Autodesk Inventor part; units mm, degrees
ref_plane "YZ Plane" through (0, 0, 0) normal (1, 0, 0) x (0, 1, 0)
ref_plane "XZ Plane" through (0, 0, 0) normal (0, 1, 0) x (-1, 0, 0)
ref_plane "XY Plane" through (0, 0, 0) normal (0, 0, 1) x (1, 0, 0)
sketch "Szkic1" plane through (0, 0, 0) normal (0, 0, 1) x (1, 0, 0)
  line L0 (3.7528, 6.5) -> (7.5056, 0)
  line L1 (7.5056, 0) -> (3.7528, -6.5)
  line L2 (3.7528, -6.5) -> (-3.7528, -6.5)
  line L3 (-3.7528, -6.5) -> (-7.5056, 0)
  line L4 (-7.5056, 0) -> (-3.7528, 6.5)
  line L5 (-3.7528, 6.5) -> (3.7528, 6.5)
  point P0 (0, 0)
  point P1 (0, 0)
  point P2 (0, 6.5)
extrude "Wyciągnięcie proste1" add sketch "Szkic1" along normal blind 5.5
sketch "Szkic2" plane through (0, 0, 5.5) normal (0, 0, 1) x (1, 0, 0)
  circle A0 centre (0, 0) radius 4
  dimension "d3" = 8
extrude "Wyciągnięcie proste2" add sketch "Szkic2" along normal blind 20
sketch "Szkic3" plane through (0, 0, 25.5) normal (0, 0, 1) x (1, 0, 0)
  circle A0 centre (0, 0) radius 4
  circle A1 centre (0, 0) radius 3.675
  dimension "d6" = 7.35
extrude "Wyciągnięcie proste3" add sketch "Szkic3" along normal blind 5 contours A1
sketch "Szkic4" plane through (0, 0, 30.5) normal (0, 0, 1) x (1, 0, 0)
  circle A0 centre (0, 0) radius 4
extrude "Wyciągnięcie proste4" add sketch "Szkic4" along normal blind 35
thread "Gwint1"
fillet "Zaokrąglenie1" radius 2 2 edges at (-3.675, 0, 25.5) (-3.675, 0, 30.5)
chamfer "Faza1" distance 0.5 angle 45 1 edges at (-4, 0, 65.5)
properties part number "COTS_GENERIC_M8_Hobbed_Bolt"
For this review, take the finished solid that the model builds, in its own axes (mm). A direction names the side the tool comes from. Round coordinates to 2 decimals unless told otherwise and drop trailing zeros. Loops run counter-clockwise (first coordinate to the right, second up) from the corner with the lowest first, then second, coordinate; pieces in that order, holes last. Notation, with made-up numbers: (33, -30) - (70, -30) arc R24 ccw to (70, -2) - close; hole circle Ø1 at (20, -2). An arc over 180 degrees is marked (long way). Put each result on its own line as item: value. Start each with the question number.
1. Consider section B-B on z = 55. State the section outline as (x, y) points, plus the area to 3 significant figures.
2. Insertion check: P1, Ø8, axis at x = -5.5, z = 25.5, coming from the +Y side; P2, Ø1, axis at x = -4, z = 55.5, coming from the +Y side; P3, Ø5, axis at x = 3.5, z = 9, coming from the -Y side. Each pin has a flat end and moves straight along its axis. Give the tip position at first contact, or say it passes through.
3. Consider section D-D on x = 5.75. State the section outline as (y, z) points, plus the area to 3 significant figures.
4. Consider section A-A on x = 0. State the section outline as (y, z) points (3 decimals).
5. For probe 1 along Z at (x, y) = (3, -4.75); probe 2 along Y at (x, z) = (-2.25, 26.5); probe 3 along X at (y, z) = (-2, 3), list the stretches that pass through material, from the lowest coordinate up. Write a range as [from, to].
6. Consider section C-C on y = 5.75. State the section outline as (x, z) points.
7. Mouldability with a two-part tool opening along Z and no side actions: class faces 1 (the flat face through (0, 0, 65.5)), 2 (the flat face through (5.66, -3.2, 2.71)), 3 (the cylindrical face through (-0.797, 3.588, 27.98)) as +Z half, -Z half, draft (parallel to the pull), parting line (faces both ways), or undercut.
8. For faces 4 (the cylindrical face through (-0.867, 3.905, 15.36)), 5 (the flat face through (-5.66, 3.2, 2.71)), list the 3-axis set-ups (+Z, -Z, +X, -X, +Y, -Y) from which the entire face can be reached by the end or side of a thin tool; tool diameter is ignored.
Result sheet:
1. outline: circle Ø8 at (0, 0)
1. area: 50.3 mm^2
2. P1: y = 3.71
2. P2: y = 1.94
2. P3: y = -3.87
3. outline: (-3.04, 0) - (3.04, 0) - (3.04, 5.5) - (-3.04, 5.5) - close
3. area: 33.4 mm^2
4. outline: (-6.5, 0) - (6.5, 0) - (6.5, 5.5) - (4, 5.5) - (4, 25.5) arc R2 cw to (3.675, 26.593) - (3.675, 29.407) arc R2 cw to (4, 30.5) - (4, 65) - (3.5, 65.5) - (-3.5, 65.5) - (-4, 65) - (-4, 30.5) arc R2 cw to (-3.675, 29.407) - (-3.675, 26.593) arc R2 cw to (-4, 25.5) - (-4, 5.5) - (-6.5, 5.5) - close
5. probe 1: [0, 5.5]
5. probe 2: [-2.91, 2.91]
5. probe 3: [-6.35, 6.35]
6. outline: (-4.19, 0) - (4.19, 0) - (4.19, 5.5) - (-4.19, 5.5) - close
7. face 1: +Z half
7. face 2: draft
7. face 3: undercut
8. face 4: +Z
8. face 5: +Z, -Z, -X, +Y
